Here's how the part is built. I have some questions about the finished solid (model axes, mm). Face numbers are marked on the shaded views. A direction names the side the tool comes from. Round coordinates to 2 decimals unless told otherwise and drop trailing zeros. One line per question, with ' | ' between items. Start each with the question number.
(1) If I drill on L1, parallel to X at y = 4.5, z = 12; L2, parallel to Z at x = 0, y = 13.1; L3, parallel to X at y = 9.5, z = 28.5, over which ranges is the centre line in solid material (lowest first)?
(2) Imagine slicing it at A-A (y = 8.5). Give the number of separate pieces and of enclosed holes in the cut face, plus the area to 3 significant figures.
(3) Thinking about a two-plate mould opening in X: for the marked faces 1, 2 and 3, which applies, pulls with the +X half, pulls with the -X half, needs draft (parallel to the pull), parting line crosses it, or undercut?
(4) For the marked faces 4, 5 and 6, which set-ups out of +Z, -Z, +X, -X, +Y, -Y let a thin tool reach every point of the face, with its end or its side?
(5) Will these pins go through, and if not, where does the flat tip stop? pin 1 (1.5 mm diameter, centred on x = 0.5, y = -7.5, fed in from -Z); pin 2 (10.5 mm diameter, centred on x = 0, z = 25.5, fed in from +Y); pin 3 (2.5 mm diameter, centred on x = 0, z = 34.3, fed in from -Y); pin 4 (6.5 mm diameter, centred on x = 1.5, z = 20, fed in from -Y).
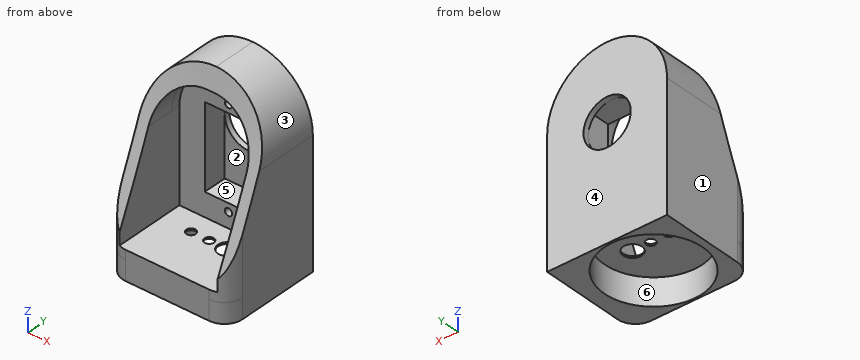
from build123d import *

# Parameters (mm, degrees)
SKETCH1_W               = 33
SKETCH1_H               = 28
BOSS_EXTRUDE1_DEPTH     = 46
CUT_EXTRUDE1_DEPTH      = 59.318093247
CUT_EXTRUDE1_DEPTH_BACK = 59.318093247
CUT_EXTRUDE2_START      = -3
CUT_EXTRUDE2_DEPTH      = 27
FILLET1_R               = 12.5
FILLET2_R               = 16.5
FILLET3_R               = 5
SKETCH4_W               = 13
SKETCH4_H               = 23
CUT_EXTRUDE3_DEPTH      = 9
SKETCH5_R               = 6.5
CUT_EXTRUDE4_DEPTH      = 56.592265809
SKETCH6_R               = 1
CUT_EXTRUDE5_DEPTH      = 8
BOSS_EXTRUDE2_DEPTH     = 5.5
SKETCH11_R              = 13.5
CUT_EXTRUDE8_DEPTH      = 7.5
SKETCH7_R               = 1.3
SKETCH7_R_2             = 2.6
CUT_EXTRUDE6_DEPTH      = 0.5
SKETCH12_R              = 1
CUT_EXTRUDE9_DEPTH      = 2.5


with BuildPart() as part:
    # Sketch1 → Boss-Extrude1 (new body)
    with BuildSketch(Plane.XY):
        Rectangle(SKETCH1_W, SKETCH1_H)
    extrude(amount=BOSS_EXTRUDE1_DEPTH)

    # Sketch2 → Cut-Extrude1 (cut, two sides: drawn at the far end of the back side and taken through both)
    with BuildSketch(Plane(origin=(16.5, 0, 0), x_dir=(0, 0, -1), z_dir=(1, 0, 0)).offset(-CUT_EXTRUDE1_DEPTH_BACK)):
        with BuildLine():
            Line((-46, -14), (-5, -14))
            add(Edge.make_bspline(
                [(-5, -14), (-31.642917286, -1.866068932), (-46, 2)],
                knots=[0, 0, 0, 1, 1, 1], degree=2))
            Line((-46, 2), (-46, -14))
        make_face()
    extrude(amount=CUT_EXTRUDE1_DEPTH + CUT_EXTRUDE1_DEPTH_BACK, mode=Mode.SUBTRACT)

    # Sketch3 → Cut-Extrude2 (cut)
    with BuildSketch(Plane(origin=(16.5, 0, 0), x_dir=(0, 0, -1), z_dir=(1, 0, 0)).offset(CUT_EXTRUDE2_START)):
        with BuildLine():
            Line((-5, -14), (-2.5, -14))
            Line((-2.5, -14), (-2.5, 3.5))
            Line((-2.5, 3.5), (-40.5, 3.5))
            Line((-40.5, 3.5), (-40.5, 0.361845))
            add(Edge.make_bspline(
                [(-5, -14), (-26.900788686, -4.025767171), (-40.5, 0.361845)],
                knots=[0, 0, 0, 1, 1, 1], degree=2))
        make_face()
    extrude(amount=-CUT_EXTRUDE2_DEPTH, mode=Mode.SUBTRACT)

    # Fillet1
    fillet1_edges = [part.edges().sort_by_distance(p)[0] for p in [
        (13.5, 1.9309225, 40.5),
        (-13.5, 1.9309225, 40.5),
    ]]
    fillet(fillet1_edges, radius=FILLET1_R)

    # Fillet2
    fillet2_edges = [part.edges().sort_by_distance(p)[0] for p in [
        (16.5, 8, 46),
        (-16.5, 8, 46),
    ]]
    fillet(fillet2_edges, radius=FILLET2_R - 0.0001)  # a hair under: the kernel refuses the full size

    # Fillet3
    fillet3_edges = [part.edges().sort_by_distance(p)[0] for p in [
        (16.5, -14, 2.5),
        (-16.5, -14, 2.5),
    ]]
    fillet(fillet3_edges, radius=FILLET3_R)

    # Sketch4 → Cut-Extrude3 (cut)
    with BuildSketch(Plane.XZ.offset(-3.5)):
        with Locations((0, 20.5)):
            Rectangle(SKETCH4_W, SKETCH4_H)
    extrude(amount=-CUT_EXTRUDE3_DEPTH, mode=Mode.SUBTRACT)

    # Sketch5 → Cut-Extrude4 (cut, through all)
    with BuildSketch(Plane.XZ.offset(-12.5)):
        with Locations((0, 25.5)):
            Circle(SKETCH5_R)
    extrude(amount=-CUT_EXTRUDE4_DEPTH, mode=Mode.SUBTRACT)

    # Sketch6 → Cut-Extrude5 (cut)
    with BuildSketch(Plane.XZ.offset(-3.5)):
        with Locations((0, 34.3)):
            Circle(SKETCH6_R)
        with Locations((0, 6.7)):
            Circle(SKETCH6_R)
    extrude(amount=-CUT_EXTRUDE5_DEPTH, mode=Mode.SUBTRACT)

    # Sketch10 → Boss-Extrude2 (add)
    with BuildSketch(Plane(origin=(0, 0, 0), x_dir=(-1, 0, 0), z_dir=(0, 0, -1))):
        with BuildLine():
            Line((-16.5, 14), (-16.5, -9))
            ThreePointArc((-16.5, -9), (-15.035533906, -12.535533906), (-11.5, -14))
            Line((-11.5, -14), (11.5, -14))
            ThreePointArc((11.5, -14), (15.035533906, -12.535533906), (16.5, -9))
            Line((16.5, -9), (16.5, 14))
            Line((16.5, 14), (-16.5, 14))
        make_face()
    extrude(amount=BOSS_EXTRUDE2_DEPTH)

    # Sketch11 → Cut-Extrude8 (cut)
    with BuildSketch(Plane(origin=(0, 0, -5.5), x_dir=(-1, 0, 0), z_dir=(0, 0, -1))):
        with Locations((1, -0.016150077)):
            Circle(SKETCH11_R)
    extrude(amount=-CUT_EXTRUDE8_DEPTH, mode=Mode.SUBTRACT)

    # Sketch7 → Cut-Extrude6 (cut)
    with BuildSketch(Plane(origin=(0, 0, 2), x_dir=(-1, 0, 0), z_dir=(0, 0, -1))):
        with Locations((5.25, 0)):
            Circle(SKETCH7_R)
        with Locations((-4.75, 0)):
            Circle(SKETCH7_R_2)
        with Locations((0.25, 0)):
            Circle(SKETCH7_R)
    extrude(amount=-CUT_EXTRUDE6_DEPTH, mode=Mode.SUBTRACT)

    # Sketch12 → Cut-Extrude9 (cut)
    with BuildSketch(Plane.XZ.offset(-3.5)):
        with BuildLine():
            Line((-13.5, 2.5), (13.5, 2.5))
            Line((13.5, 2.5), (13.5, 28))
            ThreePointArc((13.5, 28), (9.838834765, 36.838834765), (1, 40.5))
            Line((1, 40.5), (-1, 40.5))
            ThreePointArc((-1, 40.5), (-9.838834765, 36.838834765), (-13.5, 28))
            Line((-13.5, 28), (-13.5, 2.5))
        make_face()
        with Locations((0, 6.7)):
            Circle(SKETCH12_R, mode=Mode.SUBTRACT)
        Polygon((6.5, 9), (-6.5, 9), (-6.5, 32), (0, 32), (6.5, 32), align=None, mode=Mode.SUBTRACT)
        with Locations((0, 34.3)):
            Circle(SKETCH12_R, mode=Mode.SUBTRACT)
    extrude(amount=-CUT_EXTRUDE9_DEPTH, mode=Mode.SUBTRACT)


solid = part.part
Check sheet entries:
1) L1: -16.5 to -13.5, 13.5 to 16.5 | L2: 2 to 19, 32 to 46 | L3: -16.5 to -6.5, 6.5 to 16.5
2) separate pieces: 1 | enclosed holes: 3 | area: 1,120 mm^2
3) face 1: pulls with the -X half | face 2: undercut | face 3: pulls with the +X half
4) face 4: +Z, -Z, +X, -X, +Y | face 5: -Y | face 6: -Z
5) pin 1: z = 2 | pin 2: through | pin 3: y = 6 | pin 4: y = 12.5
